from build123d import *

# Parameters (mm, degrees)
F1_DEPTH = 4.826
F2_W     = 3.556
F2_H     = 1.651
F3_DEPTH = 25.4
F5_W     = 3.556
F5_H     = 1.651
F6_DEPTH = 50.8
F7_R     = 5.08
F8_R     = 5.08


with BuildPart() as f1:
    # F0 (on Front) → F1 (new body)
    with BuildSketch(Plane.XZ):
        Polygon((-25.4, 12.417778), (-41.91, -11.796889), (-41.91, -15.522222), (41.91, -15.522222), (41.91, -11.796889), (25.4, 12.417778), align=None)
        Polygon((-37.240951, -11.712222), (-23.386406, 8.607778), (23.386406, 8.607778), (37.240951, -11.712222), align=None, mode=Mode.SUBTRACT)
        Polygon((23.386406, 8.607778), (-23.386406, 8.607778), (-37.240951, -11.712222), (37.240951, -11.712222), align=None)
    extrude(amount=F1_DEPTH)

    # F2 (on Top) → F3 (cut, symmetric)
    with BuildSketch(Plane.XY):
        with Locations((11.9888, -0.8255)):
            Rectangle(F2_W, F2_H)
        Polygon((15.3543, -1.651), (13.7668, -1.651), (10.2108, -1.651), (8.6233, -1.651), (8.6233, -3.048), (15.3543, -3.048), align=None)
        with Locations((-11.9888, -0.8255)):
            Rectangle(F2_W, F2_H)
        Polygon((-10.2108, -1.651), (-13.7668, -1.651), (-15.3543, -1.651), (-15.3543, -3.048), (-8.6233, -3.048), (-8.6233, -1.651), align=None)
    extrude(amount=F3_DEPTH, both=True, mode=Mode.SUBTRACT)

    # F5 (on offset) → F6 (cut)
    with BuildSketch(Plane.XY.offset(12.7)):
        with Locations((-32.258, -0.8255)):
            Rectangle(F5_W, F5_H)
        Polygon((-30.48, -1.651), (-34.036, -1.651), (-35.6235, -1.651), (-35.6235, -3.302), (-28.8925, -3.302), (-28.8925, -1.651), align=None)
        with Locations((32.258, -0.8255)):
            Rectangle(F5_W, F5_H)
        Polygon((35.6235, -1.651), (34.036, -1.651), (30.48, -1.651), (28.8925, -1.651), (28.8925, -3.302), (35.6235, -3.302), align=None)
    extrude(amount=-F6_DEPTH, mode=Mode.SUBTRACT)

    # F7
    f7_edges = [f1.edges().sort_by_distance(p)[0] for p in [
        (-41.91, -2.413, -11.796889),
        (41.91, -2.413, -11.796889),
    ]]
    fillet(f7_edges, radius=F7_R)

    # F8
    f8_edges = [f1.edges().sort_by_distance(p)[0] for p in [
        (-25.4, -2.413, 12.417778),
        (25.4, -2.413, 12.417778),
    ]]
    fillet(f8_edges, radius=F8_R)


solid = f1.part
Can you work these out from the model? Positions are in its coordinate system, mm. A direction names the side the tool comes from. Give positions to 0.01 mm unless a question says otherwise; leave off trailing zeros. Loops run counter-clockwise (first coordinate to the right, second up) from the corner with the lowest first, then second, coordinate; pieces in that order, holes last. Notation, with made-up numbers: (54, -28.5) - (68, -28.5) arc R25 ccw to (68, -16.5) - close; hole circle Ø10 at (-28.75, 69). An arc over 180 degrees is marked (long way). One line per item, written item: value.
(1) On a 3-axis mill with a long thin cutter (end or side, diameter ignored), from which of +Z, -Z, +X, -X, +Y, -Y can I reach the whole of each face in a straight line? I mean faces 4 (the face through (-35, -1.651, -8)), 5 (the face through (-34.036, -1, -8)), 6 (the face through (25.058, -2.447, 11.845)). Say none if no direction works.
Verdict:
face 4: +Z, -Z
face 5: +Z, -Z, +Y
face 6: +Z, +X, +Y, -Y
(2) If we section it at C-C, the plane x = 37: List the corners of the cut face in (y, z) for me.
Verdict:
outline: (-4.83, -15.52) - (0, -15.52) - (0, -4.6) - (-4.83, -4.6) - close
(3) I need wall thicknesses on line 1 along X through (y, z) = (-0.35, -13); line 2 along X through (y, z) = (-1.55, 3); line 3 along X through (y, z) = (-3.15, -13). Which ranges of each line are inside material? Lowest first, please.
Verdict:
line 1: -41.9 to -34.04, -30.48 to -13.77, -10.21 to 10.21, 13.77 to 30.48, 34.04 to 41.9
line 2: -30.48 to -13.77, -10.21 to 10.21, 13.77 to 30.48
line 3: -41.9 to -35.62, -28.89 to 28.89, 35.62 to 41.9
(4) If we section it at B-B, the plane x = 11.5: List the corners of the cut face in (y, z) for me.
Verdict:
outline: (-4.83, -15.52) - (-3.05, -15.52) - (-3.05, 12.42) - (-4.83, 12.42) - close
(5) I'm going to push flat-ended pins straight in: pin 1 (0.7 mm diameter, centred on y = -2.5, z = -7, fed in from -X); pin 2 (0.7 mm diameter, centred on y = -2.5, z = -4, fed in from +X); pin 3 (0.7 mm diameter, centred on y = -2, z = -6.5, fed in from -X). Where does each tip first touch, or does it pass through?
Verdict:
pin 1: x = -38.88
pin 2: x = 36.83
pin 3: x = -38.54
(6) If we section it at A-A, the plane z = 6.5: List the corners of the cut face in (x, y) for me, plus the area to 3 significant figures.
Verdict:
outline: (-29.43, -4.83) - (29.43, -4.83) - (29.43, -3.3) - (28.89, -3.3) - (28.89, -1.65) - (29.43, -1.65) - (29.43, 0) - (13.77, 0) - (13.77, -1.65) - (15.35, -1.65) - (15.35, -3.05) - (8.62, -3.05) - (8.62, -1.65) - (10.21, -1.65) - (10.21, 0) - (-10.21, 0) - (-10.21, -1.65) - (-8.62, -1.65) - (-8.62, -3.05) - (-15.35, -3.05) - (-15.35, -1.65) - (-13.77, -1.65) - (-13.77, 0) - (-29.43, 0) - (-29.43, -1.65) - (-28.89, -1.65) - (-28.89, -3.3) - (-29.43, -3.3) - close
area: 252 mm^2
(7) If we mould it in two halves opening along Y, with no side actions, what happens to faces 1 (the face through (-22, 0, -1)), 2 (the face through (35, -1.651, -8)), 3 (the face through (13.767, -1, -2))? For each: released by +Y, released by -Y, zero draft, split by the parting line, or undercut.
Verdict:
face 1: released by +Y
face 2: undercut
face 3: zero draft
